```python
from build123d import *

# Parameters (mm, degrees)
F1_DEPTH = 1
F3_DEPTH = 1.5
F5_DEPTH = 3.001


with BuildPart() as f1:
    # F0 (on Front) → F1 (new body, symmetric)
    with BuildSketch(Plane.XZ):
        with BuildLine():
            ThreePointArc((68.7761805926, 1.2835667835), (33.7017703575, 11.9240825949), (-2.1902850165, 4.4947359819))
            ThreePointArc((-2.1902850165, 4.4947359819), (-4.3911344557, -2.3912210671), (2.5872686419, -4.278555945))
            ThreePointArc((2.5872686419, -4.278555945), (34.592048198, 5.4307267094), (67.3429144951, -1.3484207946))
            ThreePointArc((67.3429144951, -1.3484207946), (69.3173403367, -0.7173663201), (68.7761805926, 1.2835667835))
        make_face()
    extrude(amount=F1_DEPTH, both=True)

    # F2 (on Front) → F3 (join, symmetric)
    with BuildSketch(Plane.XZ):
        with BuildLine():
            ThreePointArc((16.2250227063, 7.4472055889), (9.7355101111, 5.4623847447), (3.4618675547, 2.874973571))
            ThreePointArc((3.4618675547, 2.874973571), (-4.0144119209, -2.0333462394), (4.3660093294, 1.0899369411))
            ThreePointArc((4.3660093294, 1.0899369411), (10.4167772399, 3.581978337), (16.6739491432, 5.4976668288))
            ThreePointArc((16.6739491432, 5.4976668288), (19.9548297013, 3.7331037029), (22.9673717281, 5.9245531772))
            ThreePointArc((22.9673717281, 5.9245531772), (26.5172230695, 4.7947674828), (29.0743645644, 7.5038056215))
            ThreePointArc((29.0743645644, 7.5038056215), (48.8990908767, 6.0722634585), (67.5207768882, -0.8776931178))
            ThreePointArc((67.5207768882, -0.8776931178), (68.8776931178, -0.4792231118), (68.4792231118, 0.8776931178))
            ThreePointArc((68.4792231118, 0.8776931178), (49.3016635675, 8.0314710303), (28.8856869412, 9.495447426))
            ThreePointArc((28.8856869412, 9.495447426), (25.6346945373, 11.6832952033), (22.3915524813, 9.4838272879))
            ThreePointArc((22.3915524813, 9.4838272879), (18.6203358432, 10.5485124881), (16.2250227063, 7.4472055889))
        make_face()
    extrude(amount=F3_DEPTH, both=True)

    # F4 (on face) → F5 (cut, through all)
    with BuildSketch(Plane.XZ.offset(1.5)):
        with BuildLine():
            ThreePointArc((1.0314215383, -1.7135254916), (2.5980762114, -1.5), (1.9996673749, -0.0364745084))
            ThreePointArc((1.9996673749, -0.0364745084), (1, 1.7320508076), (-1.0314215383, 1.7135254916))
            ThreePointArc((-1.0314215383, 1.7135254916), (-2.5980762114, 1.5), (-1.9996673749, 0.0364745084))
            ThreePointArc((-1.9996673749, 0.0364745084), (-1, -1.7320508076), (1.0314215383, -1.7135254916))
        make_face()
        with BuildLine():
            ThreePointArc((20.7493885716, 5.5115541672), (22.3160432446, 5.7250796588), (21.7176344082, 7.1886051503))
            ThreePointArc((21.7176344082, 7.1886051503), (20.7179670333, 8.9571304663), (18.6865454949, 8.9386051503))
            ThreePointArc((18.6865454949, 8.9386051503), (17.1198908219, 8.7250796588), (17.7182996584, 7.2615541672))
            ThreePointArc((17.7182996584, 7.2615541672), (18.7179670333, 5.4930288512), (20.7493885716, 5.5115541672))
        make_face()
        with BuildLine():
            ThreePointArc((26.6723787145, 6.4697753147), (28.2390333875, 6.6833008063), (27.640624551, 8.1468262978))
            ThreePointArc((27.640624551, 8.1468262978), (26.6409571761, 9.9153516138), (24.6095356378, 9.8968262978))
            ThreePointArc((24.6095356378, 9.8968262978), (23.0428809648, 9.6833008063), (23.6412898012, 8.2197753147))
            ThreePointArc((23.6412898012, 8.2197753147), (24.6409571761, 6.4512499987), (26.6723787145, 6.4697753147))
        make_face()
    extrude(amount=-F5_DEPTH, mode=Mode.SUBTRACT)


solid = f1.part
```
Design review of the part built by this model. Coordinates are the model's own, in mm. A direction names the side the tool comes from. Coordinates: 2 decimals unless noted, no trailing zeros. Write each loop counter-clockwise with the first axis right and the second up, starting at its lowest first coordinate (ties: lowest second). Pieces come first, ordered by that corner, then holes. Notation, with made-up numbers: M -18.75,47 L 15.25,47 A17 cw 15.25,68 Z; hole C 56,81.25 d8. An arc over 180 degrees is marked long. Answer as a JSON object with one key per item and string values.
Item 1: Add section D-D, the plane x = 63. Give the boundary of the cut face in (y, z).
Outcome:
{"outline": "M -1.5,1.38 L -1,1.38 L -1,0.58 L 1,0.58 L 1,1.38 L 1.5,1.38 L 1.5,3.57 L 1,3.57 L 1,4.44 L -1,4.44 L -1,3.57 L -1.5,3.57 Z"}
Item 2: Machinability: for faces 1 (the cylindrical face through (-4.094, -1.254, -1.868)), 2 (the cylindrical face through (34.119, -0.014, 5.408)), 3 (the cylindrical face through (9.825, 1.246, 5.494)), 4 (the cylindrical face through (1.026, -0.021, 1.717)), 5 (the cylindrical face through (48.63, 1.25, 6.13)), which of the approach directions +Z, -Z, +X, -X, +Y, -Y give a long, thin tool a straight path to every point of the face, cutting with its end or side? Answer none if there is none.
Outcome:
{"face 1": "-Y", "face 2": "-Z, +Y, -Y", "face 3": "+Z, +Y", "face 4": "+Y, -Y", "face 5": "-Z, +Y"}
Item 3: Add section A-A, the plane y = -0.35. Give the boundary of the cut face in (x, z), and give its area (3 significant figures).
Outcome:
{"outline": "M -2.19,4.49 A5 ccw long 2.59,-4.28 A67.77 cw 67.34,-1.35 A1.5 ccw 68.78,1.28 A74.27 ccw Z; hole M -2,0.04 A2 ccw 1.03,-1.71 A1 ccw long 2,-0.04 A2 ccw -1.03,1.71 A1 ccw long Z; hole M 17.72,7.26 A2 ccw 20.75,5.51 A1 ccw long 21.72,7.19 A2 ccw 18.69,8.94 A1 ccw long Z; hole M 23.64,8.22 A2 ccw 26.67,6.47 A1 ccw long 27.64,8.15 A2 ccw 24.61,9.9 A1 ccw long Z", "area": "456 mm²"}
Item 4: Wall thickness on probe 1 along X at (y, z) = (0.6, -1); probe 2 along Y at (x, z) = (46, 9); probe 3 along Z at (x, y) = (20, -1.1): over which ranges is each line inside the solid? List them lowest first.
Outcome:
{"probe 1": "-4.9 to -1.73, 2.73 to 8.69, 66.62 to 69.12", "probe 2": "-1 to 1", "probe 3": "3.74 to 5.25, 9.21 to 10.71"}
Item 5: Add section C-C, the plane x = 54. Give the boundary of the cut face in (y, z), and give its area (3 significant figures).
Outcome:
{"outline": "M -1.5,4.76 L -1,4.76 L -1,3.5 L 1,3.5 L 1,4.76 L 1.5,4.76 L 1.5,6.84 L 1,6.84 L 1,8.13 L -1,8.13 L -1,6.84 L -1.5,6.84 Z", "area": "11.3 mm²"}
Item 6: Draft analysis for pull direction X (two halves, no side actions). For faces 6 (the cylindrical face through (34.2, 0, 11.9)), 7 (the cylindrical face through (26.46, 1.25, 4.78)), 8 (the flat face through (26.6, -1.5, 5.4)), state which applies: pulls with the +X half, pulls with the -X half, needs draft (parallel to the pull), parting line crosses it, or undercut.
Outcome:
{"face 6": "parting line crosses it", "face 7": "undercut", "face 8": "needs draft"}
Item 7: Insertion check: pin 1 Ø1.2 at (x, z) = (1.73, -1) entering from +Y; pin 2 Ø8 at (x, z) = (40, 2) entering from +Y. Each pin has a flat end and moves straight along its axis. Give the tip position at first contact, or say it passes through.
Outcome:
{"pin 1": "through", "pin 2": "y = 1"}
Item 8: Add section B-B, the plane x = 0. Give the boundary of the cut face in (y, z), and give its area (3 significant figures).
Outcome:
{"outline": "M -1.5,-4.5 L -1,-4.5 L -1,-5 L 1,-5 L 1,-4.5 L 1.5,-4.5 L 1.5,-2 L -1.5,-2 Z; M -1.5,2 L 1.5,2 L 1.5,4.5 L 1,4.5 L 1,5.52 L -1,5.52 L -1,4.5 L -1.5,4.5 Z", "area": "18.0 mm²"}
